from build123d import *

# Parameters (mm, degrees)
F0_R     = 28.9
F0_R_2   = 24.25
F1_DEPTH = 33.25
F2_R     = 28.9
F3_DEPTH = 4
F4_W     = 40.4
F4_H     = 6.1
F5_DEPTH = 33.25


with BuildPart() as f1:
    # F0 (on Top) → F1 (new body)
    with BuildSketch(Plane.XY):
        Circle(F0_R)
        Circle(F0_R_2, mode=Mode.SUBTRACT)
    extrude(amount=F1_DEPTH)

    # F2 (on Top) → F3 (join)
    with BuildSketch(Plane.XY):
        Circle(F2_R)
    extrude(amount=F3_DEPTH)

    # F4 (on Top) → F5 (join, through all)
    with BuildSketch(Plane.XY):
        with BuildLine():
            Line((28.9, -73.001511), (28.9, 0))
            ThreePointArc((28.9, 0), (27.621731, -8.5), (23.9, -16.248077))
            Line((23.9, -16.248077), (23.9, -66.324389))
            Line((23.9, -66.324389), (23.9, -106.25))
            Line((23.9, -106.25), (-23.9, -106.25))
            Line((-23.9, -106.25), (-23.9, -66.324378))
            Line((-23.9, -66.324378), (-23.9, -16.248077))
            ThreePointArc((-23.9, -16.248077), (-27.621731, -8.5), (-28.9, 0))
            Line((-28.9, 0), (-28.9, -73.001511))
            Line((-28.9, -73.001511), (-28.9, -88.678621))
            Line((-28.9, -88.678621), (-28.9, -122.35))
            Line((-28.9, -122.35), (28.9, -122.35))
            Line((28.9, -122.35), (28.9, -88.678621))
            Line((28.9, -88.678621), (28.9, -73.001511))
        make_face()
        with Locations((0.05, -114.3)):
            Rectangle(F4_W, F4_H, mode=Mode.SUBTRACT)
    extrude(amount=F5_DEPTH)


solid = f1.part
Here's how the part is built. I have some questions about the finished solid (model axes, mm). A direction names the side the tool comes from. Round coordinates to 2 decimals unless told otherwise and drop trailing zeros. Write each loop counter-clockwise with the first axis right and the second up, starting at its lowest first coordinate (ties: lowest second). Pieces come first, ordered by that corner, then holes. Notation, with made-up numbers: (-11.5, 11) -> (14.5, 11) arc R32 cw to (14.5, 49) -> close; hole circle Ø5 at (21, 19.25). An arc over 180 degrees is marked (long way). One line per item, written item: value.
1) If I drill on line 1 (Y direction, x = 0, z = 15.25); line 2 (X direction, y = 0, z = 20.75); line 3 (X direction, y = -113.5, z = 22), over which ranges is the centre line in solid material (lowest first)? Write a range as [from, to].
Filled sheet:
line 1: y = [-122.35, -117.35], [-111.25, -106.25], [-28.9, -24.25], [24.25, 28.9]
line 2: x = [-28.9, -24.25], [24.25, 28.9]
line 3: x = [-28.9, -20.15], [20.25, 28.9]
2) We'd pull the mould along X, two halves only. Please class faces 4 (the face through (-28.9, -60, 16)), 5 (the face through (-0.394, -28.897, 16.392)), 6 (the face through (0, 0, 4)), 7 (the face through (0, -12, 0)): released by +X, released by -X, zero draft, split by the parting line, or undercut.
Filled sheet:
face 4: released by -X
face 5: undercut
face 6: undercut
face 7: zero draft
3) Suppose I cut it at B-B on x = 0. List the corners of the cut face in (y, z) for me.
Filled sheet:
outline: (-122.35, 0) -> (-117.35, 0) -> (-117.35, 33.25) -> (-122.35, 33.25) -> close; (-111.25, 0) -> (-106.25, 0) -> (-106.25, 33.25) -> (-111.25, 33.25) -> close; (-28.9, 0) -> (28.9, 0) -> (28.9, 33.25) -> (24.25, 33.25) -> (24.25, 4) -> (-24.25, 4) -> (-24.25, 33.25) -> (-28.9, 33.25) -> close
4) For faces 1 (the face through (0, -117.35, 16)), 2 (the face through (0.635, 28.893, 16.392)), 3 (the face through (11.19, -21.514, 18.42)), which set-ups out of +Z, -Z, +X, -X, +Y, -Y let a thin tool reach every point of the face, with its end or its side?
Filled sheet:
face 1: +Z, -Z
face 2: +Z, -Z, +Y
face 3: +Z
5) Suppose I cut it at A-A on y = -33.5. List the corners of the cut face in (x, z) for me.
Filled sheet:
outline: (-28.9, 0) -> (-23.9, 0) -> (-23.9, 33.25) -> (-28.9, 33.25) -> close; (23.9, 0) -> (28.9, 0) -> (28.9, 33.25) -> (23.9, 33.25) -> close
6) Suppose I cut it at C-C on z = 10. List the corners of the cut face in (x, y) for me.
Filled sheet:
outline: (-28.9, -122.35) -> (28.9, -122.35) -> (28.9, 0) arc R28.9 ccw to (-28.9, 0) -> close; hole circle Ø48.5 at (0, 0); hole (-23.9, -106.25) -> (23.9, -106.25) -> (23.9, -16.25) arc R28.9 cw to (-23.9, -16.25) -> close; hole (-20.15, -117.35) -> (20.25, -117.35) -> (20.25, -111.25) -> (-20.15, -111.25) -> close
7) Suppose I cut it at D-D on x = -22.5. List the corners of the cut face in (y, z) for me, plus the area to 3 significant figures.
Filled sheet:
outline: (-122.35, 0) -> (-106.25, 0) -> (-106.25, 33.25) -> (-122.35, 33.25) -> close; (-18.14, 0) -> (18.14, 0) -> (18.14, 33.25) -> (9.05, 33.25) -> (9.05, 4) -> (-9.05, 4) -> (-9.05, 33.25) -> (-18.14, 33.25) -> close
area: 1,210 mm2
8) I'm going to push flat-ended pins straight in: pin 1 Ø3 at (x, y) = (1, -18.5) entering from +Z; pin 2 Ø3 at (x, z) = (-13, 15) entering from +Y; pin 3 Ø12 at (y, z) = (6, 24) entering from +X. Where does each tip first touch, or does it pass through?
Filled sheet:
pin 1: stops at z = 4
pin 2: stops at y = 26.51
pin 3: stops at x = 28.9
